Input: part model. Units: mm. Frame: model coordinates. A direction names the side the tool comes from. Give positions to 0.01 mm unless a question says otherwise; leave off trailing zeros. Loops run counter-clockwise (first coordinate to the right, second up) from the corner with the lowest first, then second, coordinate; pieces in that order, holes last. Notation, with made-up numbers: M 71.25,-26.5 L 101.25,-26.5 A21 ccw 101.25,-11.5 Z; hole C 19.5,-34 d5. An arc over 180 degrees is marked long. Use CSV: the item, a comma, the result in double quotes. Start each with the question number.
Q1. Pull-direction query (X, two-part tool) for faces 4 (the cylindrical face through (-0.29, 7.23, 0.99)), 5 (the flat face through (-6.35, 12, 2)), 6 (the flat face through (0, 15.5, 4)), 7 (the cylindrical face through (-0.488, 17.804, 0.986)); classes: released by +X, released by -X, zero draft, split by the parting line, or undercut.
Q2. Material intervals for line 1 along Y through (x, z) = (0, 0.7); line 2 along Y through (x, z) = (-2.5, 5.25); line 3 along Z through (x, y) = (-4.5, 6.75), sorted ascending.
Q3. Section C-C, the plane z = 1.75. Output: boundary loops of the cut face in (x, y), plus the area to 3 significant figures.
Q4. Pin query (flat end, axial travel): pin 1 (3 mm diameter, centred on x = -2, z = 6, fed in from +Y); pin 2 (4 mm diameter, centred on x = 0, y = 20, fed in from -Z); pin 3 (7.5 mm diameter, centred on x = -1.5, y = 21, fed in from +Z); pin 4 (2 mm diameter, centred on x = -2, z = 5, fed in from -Y). Return the tip coordinate at first contact, or that it passes through.
Q5. Section B-B, the plane x = 0. State how many separate pieces and enclosed holes the cut face has, plus the area to 3 significant figures.
Q6. Reachability of faces 1 (the flat face through (0, 9.5, 4)), 2 (the flat face through (6.35, 12, 2)), 3 (the flat face through (-0.1, 22.4, 2)) from +Z, -Z, +X, -X, +Y, -Y: full face, straight path, thin tool, end or side. Return the list, or none.
Q7. Section A-A, the plane y = 5. Output: boundary loops of the cut face in (x, z).
from build123d import *

# Parameters (mm, degrees)
SKETCH2_W           = 12.7
SKETCH2_H           = 25
SKETCH2_R           = 2.25
BOSS_EXTRUDE1_DEPTH = 2
SKETCH3_W           = 12.7
SKETCH3_H           = 6
BOSS_EXTRUDE2_DEPTH = 7.05
CHAMFER1_SIZE       = 3


with BuildPart() as part:
    # Sketch2 → Boss-Extrude1 (new body)
    with BuildSketch(Plane.XY):
        with Locations((0, 12.5)):
            Rectangle(SKETCH2_W, SKETCH2_H)
        with Locations((0, 5)):
            Circle(SKETCH2_R, mode=Mode.SUBTRACT)
        with Locations((0, 20)):
            Circle(SKETCH2_R, mode=Mode.SUBTRACT)
    extrude(amount=BOSS_EXTRUDE1_DEPTH)

    # Sketch3 → Boss-Extrude2 (add)
    with BuildSketch(Plane.XY.offset(2)):
        with Locations((0, 12.5)):
            Rectangle(SKETCH3_W, SKETCH3_H)
    extrude(amount=BOSS_EXTRUDE2_DEPTH)

    # Chamfer1
    chamfer1_edges = [part.edges().sort_by_distance(p)[0] for p in [
        (0, 9.5, 9.05),
        (0, 15.5, 9.05),
    ]]
    chamfer(chamfer1_edges, length=CHAMFER1_SIZE - 0.0001)  # a hair under: the kernel refuses the full size


solid = part.part
A:
1,face 4,"undercut"
1,face 5,"released by -X"
1,face 6,"zero draft"
1,face 7,"undercut"
2,line 1,"0 to 2.75, 7.25 to 17.75, 22.25 to 25"
2,line 2,"9.5 to 15.5"
2,line 3,"0 to 2"
3,outline,"M -6.35,0 L 6.35,0 L 6.35,25 L -6.35,25 Z; hole C 0,5 d4.5; hole C 0,20 d4.5"
3,area,"286 mm^2"
4,pin 1,"y = 15.5"
4,pin 2,"through"
4,pin 3,"z = 2"
4,pin 4,"y = 9.5"
5,separate pieces,"3"
5,enclosed holes,"0"
5,area,"65.3 mm^2"
6,face 1,"+Z, +X, -X, -Y"
6,face 2,"+Z, -Z, +X, +Y, -Y"
6,face 3,"+Z, +X, -X, +Y"
7,outline,"M -6.35,0 L -2.25,0 L -2.25,2 L -6.35,2 Z; M 2.25,0 L 6.35,0 L 6.35,2 L 2.25,2 Z"
